```python
from build123d import *

# Parameters (mm, degrees)
F2_R     = 1.75
F3_DEPTH = 4
F4_SIZE  = 2
F5_R     = 3.25
F5_R_2   = 1.75
F6_DEPTH = 2


with BuildPart() as f3:
    # F2 (on Top) → F3 (new body)
    with BuildSketch(Plane.XY):
        Polygon((-10, -50), (0, -50), (10, -50), (10, -10), (30, -10), (30, 10), (0, 10), (-30, 10), (-30, -10), (-10, -10), align=None)
        with Locations((0, -40)):
            Circle(F2_R, mode=Mode.SUBTRACT)
        with Locations((-20, 0)):
            Circle(F2_R, mode=Mode.SUBTRACT)
        with Locations((0, -20)):
            Circle(F2_R, mode=Mode.SUBTRACT)
        Circle(F2_R, mode=Mode.SUBTRACT)
        with Locations((20, 0)):
            Circle(F2_R, mode=Mode.SUBTRACT)
    extrude(amount=F3_DEPTH)

    # F4
    f4_edges = [f3.edges().sort_by_distance(p)[0] for p in [
        (0, -50, 4),
        (10, -30, 4),
        (20, -10, 4),
        (30, 0, 4),
        (0, 10, 4),
        (-30, 0, 4),
        (-20, -10, 4),
        (-10, -30, 4),
    ]]
    chamfer(f4_edges, length=F4_SIZE)

    # F5 (on face) → F6 (cut)
    with BuildSketch(Plane.XY.offset(4)):
        with Locations((-20, 0)):
            Circle(F5_R)
        with Locations((-20, 0)):
            Circle(F5_R_2, mode=Mode.SUBTRACT)
        Circle(F5_R)
        Circle(F5_R_2, mode=Mode.SUBTRACT)
        with Locations((20, 0)):
            Circle(F5_R)
        with Locations((20, 0)):
            Circle(F5_R_2, mode=Mode.SUBTRACT)
        with Locations((0, -20)):
            Circle(F5_R)
        with Locations((0, -20)):
            Circle(F5_R_2, mode=Mode.SUBTRACT)
        with Locations((0, -40)):
            Circle(F5_R)
        with Locations((0, -40)):
            Circle(F5_R_2, mode=Mode.SUBTRACT)
    extrude(amount=-F6_DEPTH, mode=Mode.SUBTRACT)


solid = f3.part
```
Verification items for the finished model (mm, model axes). A direction names the side the tool comes from. Give positions to 0.01 mm unless a question says otherwise; leave off trailing zeros. Loops run counter-clockwise (first coordinate to the right, second up) from the corner with the lowest first, then second, coordinate; pieces in that order, holes last. Notation, with made-up numbers: M 54.5,32 L 81.5,32 A27 ccw 81.5,56 Z; hole C 40,84 d10. An arc over 180 degrees is marked long. Return JSON: item names as keys, results as strings.
1) Material ranges on L1, parallel to Y at x = 0, z = 0.75; L2, parallel to Y at x = -20, z = 0.6; L3, parallel to Y at x = -1, z = 1.25, recorded low to high. Write a range as [from, to].
Findings:
{"L1": "y = [-50, -41.75], [-38.25, -21.75], [-18.25, -1.75], [1.75, 10]", "L2": "y = [-10, -1.75], [1.75, 10]", "L3": "y = [-50, -41.44], [-38.56, -21.44], [-18.56, -1.44], [1.44, 10]"}
2) Tool access check on faces 1 (the flat face through (-19, -9, 3)), 2 (the flat face through (-20, -10, 1)), 3 (the flat face through (1.4, -1.4, 2)). Record the directions out of +Z, -Z, +X, -X, +Y, -Y that give a thin tool (end or side, any length) a straight path to the whole face; none if there is none.
Findings:
{"face 1": "+Z, -X, -Y", "face 2": "+Z, -Z, -X, -Y", "face 3": "+Z"}
3) Section check D-D, the plane x = 20. Enter the section's corners in (y, z), and give its area (3 significant figures).
Findings:
{"outline": "M -10,0 L -1.75,0 L -1.75,2 L -3.25,2 L -3.25,4 L -8,4 L -10,2 Z; M 1.75,0 L 10,0 L 10,2 L 8,4 L 3.25,4 L 3.25,2 L 1.75,2 Z", "area": "56.0 mm2"}
4) Gauge pin test, flat ends, axial feed: P1, Ø3, axis at x = 0, y = -20.5, coming from the +Z side; P2, Ø3, axis at x = 20, y = 0, coming from the -Z side; P3, Ø1, axis at y = -37, z = 1, coming from the +X side; P4, Ø1, axis at y = -21, z = 1, coming from the -X side. Record the tip position at first contact, or that the pin passes through.
Findings:
{"P1": "stops at z = 2", "P2": "passes through", "P3": "stops at x = 10", "P4": "stops at x = -10"}
5) Mould release check, pull along Y, two halves, no side actions. Record for faces 4 (the flat face through (0, 10, 1)), 5 (the cylindrical face through (16.753, 0.143, 3.014)), 6 (the flat face through (-9, -29, 3)): released by +Y, released by -Y, zero draft, split by the parting line, or undercut.
Findings:
{"face 4": "released by +Y", "face 5": "undercut", "face 6": "zero draft"}
6) Section check C-C, the plane z = 1.35. Enter the section's corners in (x, y).
Findings:
{"outline": "M -30,-10 L -10,-10 L -10,-50 L 10,-50 L 10,-10 L 30,-10 L 30,10 L -30,10 Z; hole C -20,0 d3.5; hole C 0,-40 d3.5; hole C 0,-20 d3.5; hole C 0,0 d3.5; hole C 20,0 d3.5"}
7) Section check A-A, the plane y = 0. Count the separate pieces of the cut face and the enclosed holes in it, and give its area (3 significant figures).
Findings:
{"separate pieces": "4", "enclosed holes": "0", "area": "176 mm2"}
